Could you check a few things on this model? Use its own coordinates, in mm. A direction names the side the tool comes from. Coordinates: 2 decimals unless noted, no trailing zeros. Write each loop counter-clockwise with the first axis right and the second up, starting at its lowest first coordinate (ties: lowest second). Pieces come first, ordered by that corner, then holes.
Item 1: Which directions (+Z, -Z, +X, -X, +Y, -Y) give clear straight access to the entire face, cutting with the end or side of a thin tool? Please do faces 4 (the flat face through (-8, 8, 13.5)), 5 (the flat face through (57, 15, -11.5)), 6 (the flat face through (12, 16, 15)).
Item 2: Thinking about a two-plate mould opening in X: for faces 1 (the flat face through (58.5, 8, 0)), 2 (the flat face through (14.5, 8, 2)), 3 (the cylindrical face through (57.51, 12.6, -4.07)), which applies, +X half, -X half, draft (parallel to the pull), parting line (faces both ways), or undercut?
Item 3: I want a section at C-C on z = -10. Please give me the cut outline in (x, y).
Item 4: If I drill on probe 1 along X at (y, z) = (14.25, 0.5); probe 2 along Z at (x, y) = (1, 12); probe 3 along X at (y, z) = (8.75, -4.5), over which ranges is the centre line in solid material (lowest first)?
Item 5: I want a section at D-D on y = 4. Please give me the cut outline in (x, z), then the cut area to 3 significant figures.
Item 6: I want a section at A-A on x = -35.5. Please give me the cut outline in (y, z), then the cut area to 3 significant figures.
Item 7: For P1, Ø4, axis at x = -13.5, z = 10.5, coming from the +Y side, with a flat end and sliding along its axis, tell me the tip position at first contact or that it passes through.
Item 8: I want a section at B-B on z = 22.5. Please give me the cut outline in (x, y).
Autodesk Inventor part; units mm, degrees
ref_plane "YZ Plane" through (0, 0, 0) normal (1, 0, 0) x (0, 1, 0)
ref_plane "XZ Plane" through (0, 0, 0) normal (0, 1, 0) x (-1, 0, 0)
ref_plane "XY Plane" through (0, 0, 0) normal (0, 0, 1) x (1, 0, 0)
sketch "Sketch1" plane through (0, 0, 0) normal (0, 1, 0) x (-1, 0, 0)
  line L0 (-58.5, 29.5) -> (42.5, 29.5)
  line L1 (42.5, 29.5) -> (42.5, -29.5)
  line L2 (42.5, -29.5) -> (-58.5, -29.5)
  line L3 (-58.5, -29.5) -> (-58.5, 29.5)
  line L4 (0, 10) -> (2.5, 10)
  line L5 (2.5, 10) -> (12.5, 10)
  line L6 (-14.5, 20.5) -> (-56.5, 20.5)
  line L7 (-56.5, 20.5) -> (-56.5, -0.5)
  line L8 (-56.5, -0.5) -> (-14.5, -0.5)
  line L9 (-14.5, -0.5) -> (-14.5, 20.5)
  line L10 (12.5, 13.5) -> (12.5, 6.5)
  line L11 (12.5, 6.5) -> (2.5, 6.5)
  line L12 (12.5, 13.5) -> (2.5, 13.5)
  line L13 (40.5, 27.5) -> (12.5, 27.5)
  line L14 (12.5, 27.5) -> (12.5, -27.5)
  line L15 (12.5, -27.5) -> (40.5, -27.5)
  line L16 (40.5, -27.5) -> (40.5, 27.5)
  line L17 (12.5, 27.5) -> (12.5, 29.5)
  line L18 (12.5, -27.5) -> (12.5, -29.5)
  line L19 (0, 0) -> (0, 10)
  line L20 (2.5, 13.5) -> (2.5, 6.5)
  line L21 (2.5, 14.5) -> (2.5, 5.5)
  line L22 (2.5, 5.5) -> (-14.5, 5.5)
  line L23 (2.5, 14.5) -> (-14.5, 14.5)
  line L24 (12.5, 0) -> (0, 0)
  line L25 (-56.5, -0.5) -> (12.5, -0.5)
  line L26 (12.5, -0.5) -> (12.5, -27.5)
  line L27 (12.5, -27.5) -> (-56.5, -27.5)
  line L28 (-56.5, -27.5) -> (-56.5, -0.5)
  line L29 (2.5, 5.5) -> (2.5, 0)
  point P0 (-8, 29.5)
  point P1 (0, 5.5)
  dimension "d2" = 2.5
  dimension "d3" = 10
  dimension "d4" = 7
  dimension "d5" = 21
  dimension "d6" = 42
  dimension "d9" = 28
  dimension "d10" = 55
  dimension "d13" = 10
  dimension "d14" = 9
  dimension "d15" = 17
  dimension "d16" = 2
  dimension "d17" = 2
  dimension "d20" = 2
  dimension "d28" = 101
  dimension "d29" = 59
  dimension "d34" = 42
  dimension "d35" = 27
  dimension "d37" = 12.5
sketch "Sketch2" plane through (0, 0, 0) normal (0, 1, 0) x (-1, 0, 0)
  line L0 (0, 0) -> (12.5, 0)
  line L1 (40.5, -27.5) -> (-56.5, -27.5)
  line L2 (12.5, 0) -> (12.5, -27.5)
  line L3 (12.5, 0) -> (0, 0)
  line L4 (0, 0) -> (0, -27.5)
  line L5 (0, -27.5) -> (12.5, -27.5)
  line L6 (12.5, -27.5) -> (12.5, 0)
  dimension "d36" = 56.5
extrude "Extrusion5" add sketch "Sketch2" along normal blind 10
extrude "Extrusion6" add sketch "Sketch1" along normal blind 16 contours L0 L17 L14 L12 L21 L23 L9 L6 L7 L28 L27 L18 L2 L3 | L0 L1 L2 L18 L15 L16 L13 L17 | L25 L9 L22 L19 L24 L14 | L14 L24 L29 L21 L11 | L24 L19 L22 L29
sketch "Sketch3" plane through (0, 16, 0) normal (0, 1, 0) x (1, 0, 0)
  line L0 (56.5, 3.5) -> (56.5, 7.5)
  line L1 (56.5, 7.5) -> (56.5, 11.5)
  line L2 (56.5, 11.5) -> (56.5, 15.5)
  line L3 (56.5, 15.5) -> (56.5, 19.5)
  line L4 (56.5, 19.5) -> (56.5, 23.5)
  line L5 (56.5, 23.5) -> (56.5, 27.5)
  line L6 (58.5, -29.5) -> (58.5, 29.5)
  line L7 (56.5, 23.5) -> (58.5, 23.5)
  line L8 (58.5, -29.5) -> (58.5, 29.5)
  line L9 (56.5, 19.5) -> (58.5, 19.5)
  line L10 (56.5, 15.5) -> (58.5, 15.5)
  line L11 (56.5, 11.5) -> (58.5, 11.5)
  line L12 (56.5, 7.5) -> (58.5, 7.5)
  line L13 (56.5, 3.5) -> (58.5, 3.5)
  point P0 (0, 0)
  dimension "d30" = 4
extrude "Extrusion7" cut sketch "Sketch3" against normal blind 4 contours L0 L12 L6 L13 | L2 L10 L6 L11 | L4 L7 L6 L9
fillet "Fillet1" radius 2 6 edges at (57.5, 12, -3.5) (57.5, 12, -11.5) (57.5, 12, -19.5) (57.5, 12, -23.5) (57.5, 12, -15.5) (57.5, 12, -7.5)
properties part number "Lag4"
Response values:
1. face 4: +Y, -Y
1. face 5: +X, +Y
1. face 6: +Z, -Z, +X, -X, +Y
2. face 1: +X half
2. face 2: undercut
2. face 3: draft
3. outline: (-42.5, 0) - (-40.5, 0) - (-40.5, 16) - (-42.5, 16) - close; (-12.5, 0) - (0, 0) - (0, 10) - (-12.5, 10) - close; (56.5, 0) - (58.5, 0) - (58.5, 16) - (56.5, 16) - close
4. probe 1: x = -42.5 to -40.5, -12.5 to 14.5, 56.5 to 58.5
4. probe 2: z = -29.5 to -27.5, -0.5 to 5.5, 14.5 to 29.5
4. probe 3: x = -42.5 to -40.5, -12.5 to 0, 56.5 to 58.5
5. outline: (-42.5, -29.5) - (58.5, -29.5) - (58.5, 29.5) - (-42.5, 29.5) - close; hole (-40.5, -27.5) - (-12.5, -27.5) - (-12.5, 6.5) - (-2.5, 6.5) - (-2.5, 5.5) - (14.5, 5.5) - (14.5, -0.5) - (0, -0.5) - (0, -27.5) - (56.5, -27.5) - (56.5, 20.5) - (14.5, 20.5) - (14.5, 14.5) - (-2.5, 14.5) - (-2.5, 13.5) - (-12.5, 13.5) - (-12.5, 27.5) - (-40.5, 27.5) - close
5. area: 1,790 mm2
6. outline: (0, -29.5) - (16, -29.5) - (16, -27.5) - (0, -27.5) - close; (0, 27.5) - (16, 27.5) - (16, 29.5) - (0, 29.5) - close
6. area: 64.0 mm2
7. P1: passes through
8. outline: (-42.5, 0) - (-40.5, 0) - (-40.5, 16) - (-42.5, 16) - close; (-12.5, 0) - (58.5, 0) - (58.5, 16) - (-12.5, 16) - close
